Work out the finished part from the listing and answer in its coordinate system (mm). A direction names the side the tool comes from. Round coordinates to 2 decimals unless told otherwise and drop trailing zeros. Order: outer loops, then holes, each group sorted by start corner. A loop starts at its lowest first (then second) coordinate and runs counter-clockwise, first axis right, second up. Notation, with made-up numbers: (72.5, -32) - (101.5, -32) arc R25 cw to (101.5, -4) - close; hole circle Ø1 at (-3, 5). An arc over 180 degrees is marked (long way). Answer in a Markdown table with one row per item.
Autodesk Inventor part; units mm, degrees
ref_plane "YZ Plane" through (0, 0, 0) normal (1, 0, 0) x (0, 1, 0)
ref_plane "XZ Plane" through (0, 0, 0) normal (0, 1, 0) x (-1, 0, 0)
ref_plane "XY Plane" through (0, 0, 0) normal (0, 0, 1) x (1, 0, 0)
sketch "草图1" plane through (0, 0, 0) normal (0, 1, 0) x (-1, 0, 0)
  line L0 (-16, 26) -> (16, 26)
  line L1 (16, 26) -> (16, -26)
  line L2 (16, -26) -> (-16, -26)
  line L3 (-16, -26) -> (-16, 26)
  line L4 (-16, 26) -> (16, -26) construction
  line L5 (16, 26) -> (-16, -26) construction
  point P0 (0, 0)
  dimension "d0" = 52
  dimension "d1" = 32
extrude "拉伸1" add sketch "草图1" along normal blind 8
sketch "草图2" plane through (0, 8, 0) normal (0, 1, 0) x (1, 0, 0)
  line L0 (13, -14) -> (-13, -14)
  line L1 (-13, -14) -> (-13, 14)
  line L2 (-13, 14) -> (13, 14)
  line L3 (13, 14) -> (13, -14)
  line L4 (13, -14) -> (-13, 14) construction
  line L5 (-13, -14) -> (13, 14) construction
  point P0 (0, 0)
  dimension "d4" = 28
  dimension "d5" = 26
extrude "拉伸2" add sketch "草图2" along normal blind 18
sketch "草图3" plane through (16, 0, 26) normal (1, 0, 0) x (0, 0, -1)
  line L0 (10, -2) -> (42, -2)
  line L1 (42, -2) -> (42, 2)
  line L2 (42, 2) -> (10, 2)
  line L3 (10, 2) -> (10, -2)
  line L4 (10, -2) -> (42, 2) construction
  line L5 (42, -2) -> (10, 2) construction
  line L6 (52, 0) -> (0, 0)
  point P0 (26, 0)
  dimension "d8" = 2
  dimension "d9" = 32
extrude "拉伸3" cut sketch "草图3" against normal through all
sketch "草图4" plane through (16, 0, -26) normal (1, 0, 0) x (0, 0, -1)
  line L0 (-40, 26) -> (-12, 26) construction
  line L1 (-26, 26) -> (-26, 12) construction
  circle A0 centre (-26, 12) radius 8
  point P0 (-26, 0)
  dimension "d12" = 14
  dimension "d13" = 16
extrude "拉伸4" cut sketch "草图4" against normal up to surface (3 mm away)
sketch "草图5" plane through (0, 8, 0) normal (0, 1, 0) x (1, 0, 0)
  line L0 (10, -21) -> (-10, -21) construction
  line L1 (-10, -21) -> (-10, 21) construction
  line L2 (-10, 21) -> (10, 21) construction
  line L3 (10, 21) -> (10, -21) construction
  line L4 (10, -21) -> (-10, 21) construction
  line L5 (-10, -21) -> (10, 21) construction
  circle A0 centre (-10, -21) radius 3
  circle A1 centre (-10, 21) radius 3
  circle A2 centre (10, 21) radius 3
  circle A3 centre (10, -21) radius 3
  line L6 (16, -26) -> (-16, -26)
  point P0 (0, 0)
  dimension "d16" = 6
  dimension "d18" = 20
  dimension "d19" = 5
extrude "拉伸5" cut sketch "草图5" against normal blind 18
sketch "草图6" plane through (0, 0, 0) normal (0, -1, 0) x (1, 0, 0)
  line L0 (-10, 10) -> (10, 10)
  line L1 (10, 10) -> (10, -10)
  line L2 (10, -10) -> (-10, -10)
  line L3 (-10, -10) -> (-10, 10)
  line L4 (-10, 10) -> (10, -10) construction
  line L5 (10, 10) -> (-10, -10) construction
  point P0 (0, 0)
  dimension "d22" = 20
  dimension "d23" = 20
extrude "拉伸6" cut sketch "草图6" against normal blind 24
sketch "草图7" plane through (13, 8, -14) normal (1, 0, 0) x (0, 0, -1)
  line L0 (0, 18) -> (-28, 18) construction
  line L1 (-14, 18) -> (-14, 0) construction
  circle A0 centre (-14, 0) radius 2
  point P0 (-14, -8)
  dimension "d26" = 18
  dimension "d27" = 4
extrude "拉伸7" cut sketch "草图7" against normal up to surface (3 mm away)
sketch "草图8" plane through (0, 26, 0) normal (0, 1, 0) x (1, 0, 0)
  circle A0 centre (0, 0) radius 8
  dimension "d30" = 16
extrude "拉伸8" add sketch "草图8" along normal blind 2 and the other way blind 12
sketch "草图9" plane through (0, 28, 0) normal (0, 1, 0) x (1, 0, 0)
  circle A0 centre (0, 0) radius 5
  dimension "d35" = 10
extrude "拉伸9" cut sketch "草图9" against normal blind 12
sketch "草图10" plane through (0, 16, 0) normal (0, 1, 0) x (1, 0, 0)
  circle A0 centre (0, 0) radius 3
  dimension "d38" = 6
extrude "拉伸10" cut sketch "草图10" against normal blind 12
properties part number "模型3"
1) The mould has two halves that part along Z. Classify faces 1 (the face through (0, 4, 26)), 2 (the face through (0, 1, 16)), 3 (the face through (-13, 17, 0)): released by +Z, released by -Z, zero draft, split by the parting line, or undercut.
Filled in:
| item | result |
|---|---|
| face 1 | released by +Z |
| face 2 | undercut |
| face 3 | zero draft |
2) Find section D-D, the plane y = 14.75. Give the vertices of the cut face in (x, z).
Filled in:
| item | result |
|---|---|
| outline | (-13, -14) - (13, -14) - (13, 14) - (-13, 14) - close; circle Ø16 at (0, 0); hole (-10, -10) - (10, -10) - (10, 10) - (-10, 10) - close; hole circle Ø6 at (0, 0) |
3) Find section C-C, the plane z = 21. Give the vertices of the cut face in (x, y).
Filled in:
| item | result |
|---|---|
| outline | (-16, 0) - (-13, 0) - (-13, 8) - (-16, 8) - close; (-7, 0) - (7, 0) - (7, 8) - (-7, 8) - close; (13, 0) - (16, 0) - (16, 8) - (13, 8) - close |
4) Find section A-A, the plane y = 18. Give the vertices of the cut face in (x, z), then the cut area to 3 significant figures.
Filled in:
| item | result |
|---|---|
| outline | (-13, -14) - (13, -14) - (13, 14) - (-13, 14) - close; circle Ø16 at (0, 0); hole (-10, -10) - (10, -10) - (10, 10) - (-10, 10) - close; hole circle Ø10 at (0, 0) |
| area | 451 mm^2 |
5) Find the intervals of material crossed by probe 1 along X at (y, z) = (14.55, 0); probe 2 along X at (y, z) = (3, 21); probe 3 along X at (y, z) = (20.75, 0), in increasing order. Write a range as from..to.
Filled in:
| item | result |
|---|---|
| probe 1 | x = -13..-10, -8..-3, 3..8, 10..13 |
| probe 2 | x = -16..-13, -7..7, 13..16 |
| probe 3 | x = -13..-10, -8..-5, 5..8, 10..13 |
6) Which of the six approach directions +Z, -Z, +X, -X, +Y, -Y give full straight-line access (tool end or side, diameter ignored) to faces 4 (the face through (0, 1, -16)), 5 (the face through (-6, 26, 6)), 6 (the face through (3.4, 14, -0.1)), 7 (the face through (0, 17, 14))?
Filled in:
| item | result |
|---|---|
| face 4 | +X, -X, -Y |
| face 5 | +Y |
| face 6 | -Y |
| face 7 | +Z, +X, -X, +Y |
7) Each of these flat-tipped pins is pushed along its axis until it touches: pin 1 (8 mm diameter, centred on x = -0.5, z = 4, fed in from -Y); pin 2 (6.5 mm diameter, centred on y = 14, z = 1, fed in from +X); pin 3 (3 mm diameter, centred on x = 10, z = -8.5, fed in from -Y). Where does it stop, or does it pass through?
Filled in:
| item | result |
|---|---|
| pin 1 | stops at y = 14 |
| pin 2 | stops at x = 13 |
| pin 3 | stops at y = 2 |
